from build123d import *

# Parameters (mm, degrees)
SKETCH1_W                      = 32
SKETCH1_H                      = 5
BASE_FLANGE1_DEPTH             = 1
EDGE_FLANGE1_STRIP_W           = 5.4732
EDGE_FLANGE1_STRIP_H           = 1
EDGE_FLANGE1_STRIP_CUT_DEPTH   = 5
EDGE_FLANGE1_STRIP_2_W         = 5.4732
EDGE_FLANGE1_STRIP_2_H         = 1
EDGE_FLANGE1_STRIP_CUT_2_DEPTH = 5
EDGE_FLANGE1_DEPTH             = 5
EDGE_FLANGE1_BEND_DEPTH        = 5
BOSS_EXTRUDE1_DEPTH            = 1
BOSS_EXTRUDE2_DEPTH            = 1


# Sheet-metal steps are written as plain solids
with BuildPart() as part:
    # Sketch1 → Base-Flange1 (new body)
    with BuildSketch(Plane.XY):
        Rectangle(SKETCH1_W, SKETCH1_H)
    extrude(amount=-BASE_FLANGE1_DEPTH)

    # Edge-Flange1 strip (across the edge) → Edge-Flange1 strip cut (cut)
    with BuildSketch(Plane(origin=(-16, 2.5, 0), x_dir=(1, 0, 0), z_dir=(0, -1, 0))):
        with Locations((-1, -0.5)):
            Rectangle(EDGE_FLANGE1_STRIP_W, EDGE_FLANGE1_STRIP_H)
    extrude(amount=EDGE_FLANGE1_STRIP_CUT_DEPTH, mode=Mode.SUBTRACT)

    # Edge-Flange1 strip 2 (across the edge) → Edge-Flange1 strip cut 2 (cut)
    with BuildSketch(Plane(origin=(16, -2.5, 0), x_dir=(-1, 0, 0), z_dir=(0, 1, 0))):
        with Locations((-1, -0.5)):
            Rectangle(EDGE_FLANGE1_STRIP_2_W, EDGE_FLANGE1_STRIP_2_H)
    extrude(amount=EDGE_FLANGE1_STRIP_CUT_2_DEPTH, mode=Mode.SUBTRACT)

    # Edge-Flange1 section (across the edge) → Edge-Flange1 (add)
    with BuildSketch(Plane(origin=(-16, 2.5, 0), x_dir=(1, 0, 0), z_dir=(0, -1, 0))):
        with BuildLine():
            Line((0, 0.7366), (0, 23.7366))
            Line((0, 23.7366), (1, 23.7366))
            Line((1, 23.7366), (1, 0.7366))
            ThreePointArc((1, 0.7366), (1.215745145, 0.215745145), (1.7366, 0))
            Line((1.7366, 0), (1.7366, -1))
            ThreePointArc((1.7366, -1), (0.508638364, -0.491361636), (0, 0.7366))
        make_face()
    extrude(amount=EDGE_FLANGE1_DEPTH)

    # Edge-Flange1 section 2 (across the edge) → Edge-Flange1 bend (add)
    with BuildSketch(Plane(origin=(16, -2.5, 0), x_dir=(-1, 0, 0), z_dir=(0, 1, 0))):
        with BuildLine():
            Line((0, 0.7366), (0, 23.7366))
            Line((0, 23.7366), (1, 23.7366))
            Line((1, 23.7366), (1, 0.7366))
            ThreePointArc((1, 0.7366), (1.215745145, 0.215745145), (1.7366, 0))
            Line((1.7366, 0), (1.7366, -1))
            ThreePointArc((1.7366, -1), (0.508638364, -0.491361636), (0, 0.7366))
        make_face()
    extrude(amount=EDGE_FLANGE1_BEND_DEPTH)

    # Sketch12 → Boss-Extrude1 (add)
    with BuildSketch(Plane(origin=(16, 0, 0), x_dir=(0, 0, -1), z_dir=(1, 0, 0))):
        Polygon((-19.622935429, -0.632906062), (-19.686371165, 0.74277998), (-20.909468094, 1.375686043), (-22.069129286, 0.632906062), (-22.00569355, -0.74277998), (-20.782596622, -1.375686043), align=None)
    extrude(amount=BOSS_EXTRUDE1_DEPTH)

    # Sketch13 → Boss-Extrude2 (add)
    with BuildSketch(Plane.ZY.offset(16)):
        Polygon((22.141401041, -0.649858365), (21.962250454, 0.960156284), (20.478361573, 1.61001465), (19.17362328, 0.649858365), (19.352773867, -0.960156284), (20.836662748, -1.61001465), align=None)
    extrude(amount=BOSS_EXTRUDE2_DEPTH)


solid = part.part
The model under review builds one solid part; all positions refer to its coordinate system, in mm. A direction names the side the tool comes from. Give positions to 0.01 mm unless a question says otherwise; leave off trailing zeros. Write each loop counter-clockwise with the first axis right and the second up, starting at its lowest first coordinate (ties: lowest second). Pieces come first, ordered by that corner, then holes.
1. Add section B-B, the plane y = 2. Write out the cut boundary in (x, z).
2. Add section A-A, the plane z = 5.75. Write out the cut boundary in (x, y), plus the area to 3 significant figures.
3. Add section C-C, the plane x = 13. Write out the cut boundary in (y, z).
4. Wall thickness on L1, parallel to X at y = -1.85, z = 18.5; L2, parallel to Z at x = -3.5, y = 1.1; L3, parallel to X at y = 0.4, z = 20.75: over which ranges is each line inside the solid? List them lowest first.
5. Draft analysis for pull direction X (two halves, no side actions). For faces 4 (the flat face through (-15, 0, 12)), 5 (the flat face through (-16.49, -1.28, 20.08)), 6 (the flat face through (-16, 0, 12)), state which applies: +X half, -X half, draft (parallel to the pull), parting line (faces both ways), or undercut.
6. For P1, Ø1.5, axis at y = -1, z = 7.5, coming from the +X side; P2, Ø3, axis at y = 0.5, z = 4.5, coming from the -X side; P3, Ø1.5, axis at x = -13.5, y = 0, coming from the +Z side, all flat-tipped, find the tip position at first contact; note any pin that passes through.
7. Add section D-D, the plane y = 0.25. Write out the cut boundary in (x, z), plus the area to 3 significant figures.
8. Tool access review of faces 1 (the flat face through (0, 0, 0)), 2 (the flat face through (16.493, -1.055, 21.403)), 3 (the flat face through (16.493, 1.055, 20.289)): name each direction out of +Z, -Z, +X, -X, +Y, -Y from which nothing blocks a thin tool from reaching the whole face with its end or side.
Worked answers:
1. outline: (-16, 0.74) arc R1.74 ccw to (-14.26, -1) - (14.26, -1) arc R1.74 ccw to (16, 0.74) - (16, 23.74) - (15, 23.74) - (15, 0.74) arc R0.74 cw to (14.26, 0) - (-14.26, 0) arc R0.74 cw to (-15, 0.74) - (-15, 23.74) - (-16, 23.74) - close
2. outline: (-16, -2.5) - (-15, -2.5) - (-15, 2.5) - (-16, 2.5) - close; (15, -2.5) - (16, -2.5) - (16, 2.5) - (15, 2.5) - close
2. area: 10.0 mm2
3. outline: (-2.5, -1) - (2.5, -1) - (2.5, 0) - (-2.5, 0) - close
4. L1: x = -16 to -15, 15 to 16
4. L2: z = -1 to 0
4. L3: x = -17 to -15, 15 to 17
5. face 4: undercut
5. face 5: draft
5. face 6: -X half
6. P1: stops at x = 16
6. P2: stops at x = -16
6. P3: stops at z = 0
7. outline: (-17, 19.22) - (-16, 19.22) - (-16, 0.74) arc R1.74 ccw to (-14.26, -1) - (14.26, -1) arc R1.74 ccw to (16, 0.74) - (16, 19.66) - (17, 19.66) - (17, 22.05) - (16, 22.05) - (16, 23.74) - (15, 23.74) - (15, 0.74) arc R0.74 cw to (14.26, 0) - (-14.26, 0) arc R0.74 cw to (-15, 0.74) - (-15, 23.74) - (-16, 23.74) - (-16, 22.04) - (-17, 22.04) - close
7. area: 83.6 mm2
8. face 1: +Z, +Y, -Y
8. face 2: +Z, +X, -Y
8. face 3: -Z, +X, +Y
